Design review of the part built by this model. Coordinates are the model's own, in mm. A direction names the side the tool comes from. Round coordinates to 2 decimals unless told otherwise and drop trailing zeros. Loops run counter-clockwise (first coordinate to the right, second up) from the corner with the lowest first, then second, coordinate; pieces in that order, holes last. Notation, with made-up numbers: (-39.5, -7) - (4.5, -7) arc R26 cw to (4.5, 29) - close; hole circle Ø2 at (-14, 64). An arc over 180 degrees is marked (long way). Answer as CSV lines item,"result". Start each with the question number.
(1) Consider section C-C (x = 9.75). Give the boundary of the cut face in (y, z).
(2) For P1, Ø2, axis at y = -31, z = -8.5, coming from the +X side; P2, Ø6.5, axis at x = 11, z = -7.5, coming from the +Y side; P3, Ø10, axis at x = 15, y = -48.5, coming from the -Z side, all flat-tipped, find the tip position at first contact; note any pin that passes through.
(3) Consider section A-A (x = 15.4). Give the boundary of the cut face in (y, z).
(4) Mouldability with a two-part tool opening along X and no side actions: class faces 1 (the flat face through (14, -52.511, -3)), 2 (the cylindrical face through (3.417, -42.54, -3.588)), 3 (the flat face through (0, -20, -10)) as released by +X, released by -X, zero draft, split by the parting line, or undercut.
(5) Consider section B-B (y = -42.8). Give the boundary of the cut face in (x, z) (3 decimals), and give its area (3 significant figures).
(6) Wall thickness on L1, parallel to X at y = -42.8, z = -3.25 (3 decimals); L2, parallel to Y at x = 15.4, z = -2.75; L3, parallel to Y at x = 10.75, z = -5: over which ranges is each line inside the solid? List them lowest first.
(7) For faces 4 (the flat face through (-2, -20, 0)), 5 (the flat face through (13, 6, -6.35)), 6 (the flat face through (14, 12.7, -3)), 7 (the flat face through (-2, -21, -19.05)), 8 (the flat face through (10, 0, -3)), list the 3-axis set-ups (+Z, -Z, +X, -X, +Y, -Y) from which the entire face can be reached by the end or side of a thin tool; tool diameter is ignored.
(8) Consider section D-D (z = -3.5). Give the boundary of the cut face in (x, y) (3 decimals).
Autodesk Inventor part; units mm, degrees
ref_plane "YZ Plane" through (0, 0, 0) normal (1, 0, 0) x (0, 1, 0)
ref_plane "XZ Plane" through (0, 0, 0) normal (0, 1, 0) x (-1, 0, 0)
ref_plane "XY Plane" through (0, 0, 0) normal (0, 0, 1) x (1, 0, 0)
sketch "Sketch1" plane through (0, 0, 0) normal (0, 0, 1) x (1, 0, 0)
  line L0 (0, 0) -> (20.8, 0)
  line L1 (20.8, 0) -> (20.8, 12.7)
  line L2 (20.8, 12.7) -> (0, 12.7)
  line L3 (0, 12.7) -> (0, 0)
  line L4 (0, -39.8112) -> (20.8, -39.8112)
  line L5 (20.8, -39.8112) -> (20.8, -52.5112)
  line L6 (20.8, -52.5112) -> (0, -52.5112)
  line L7 (0, -52.5112) -> (0, -39.8112)
  line L8 (10.4, 12.7) -> (10.4, 0)
  point P0 (5.4, 3)
  dimension "d0" = 20.8
  dimension "d1" = 12.7
  dimension "d2" = 39.8112
  dimension "d33" = 3
  dimension "d34" = 5
  dimension "d41" = 10.4
extrude "Extrusion1" add sketch "Sketch1" against normal blind 6.35
hole "Hole3" at (5.4, 3, 0) direction (0, 0, -1) diameter 4 depth 25.4
pattern_linear "Rectangular Pattern1" count 2 spacing 10 along (1, 0, 0) count 2 spacing 45.8 along (0, -1, 0) of "Hole3"
sketch "Sketch3" plane through (0, 0, 0) normal (-1, 0, 0) x (0, 0, 1)
  line L0 (0, 12.7) -> (0, 0)
  line L1 (-19.05, 24.4) -> (0, 24.4)
  line L2 (0, 24.4) -> (0, -65.2112)
  line L3 (0, -65.2112) -> (-19.05, -65.2112)
  line L4 (-19.05, -65.2112) -> (-19.05, 24.4)
  line L5 (0, -39.8112) -> (-6.35, -39.8112)
  dimension "d42" = 19.05
  dimension "ServoMountLength" = 89.6112
  dimension "d45" = 25.4
extrude "Extrusion2" add sketch "Sketch3" along normal blind 3.175
fillet "Fillet1" radius 6.35 4 edges at (0, 6.35, -6.35) (0, 12.7, -3.175) (0, -46.1612, -6.35) (0, -52.5112, -3.175)
equation "\"d0\" = ServoWidth + ServoTolerance"
equation "\"d2\" = ServoLength + ServoTolerance"
equation "\"d41\" = 0.5 * ServoTolerance + 0.5 * ServoWidth"
equation "\"d37\" = ServoScrewSpacing"
equation "\"d40\" = ServoScrewSpacingLength"
equation "\"ServoTolerance\" = 1"
properties part number "ServoMount" material "ABS Plastic"
Determined:
1,outline,"(-52.51, -6.35) - (-39.81, -6.35) - (-39.81, 0) - (-52.51, 0) - close; (0, -6.35) - (12.7, -6.35) - (12.7, 0) - (0, 0) - close"
2,P1,"stops at x = 0"
2,P2,"stops at y = 12.7"
2,P3,"stops at z = -6.35"
3,outline,"(-52.51, -6.35) - (-44.8, -6.35) - (-44.8, 0) - (-52.51, 0) - close; (-40.8, -6.35) - (-39.81, -6.35) - (-39.81, 0) - (-40.8, 0) - close; (0, -6.35) - (1, -6.35) - (1, 0) - (0, 0) - close; (5, -6.35) - (12.7, -6.35) - (12.7, 0) - (5, 0) - close"
4,face 1,"zero draft"
4,face 2,"undercut"
4,face 3,"released by +X"
5,outline,"(-3.175, -19.05) - (0, -19.05) - (0, -12.7) arc R6.35 cw to (3.4, -7.077) - (3.4, 0) - (-3.175, 0) - close; (7.4, -6.35) - (13.4, -6.35) - (13.4, 0) - (7.4, 0) - close; (17.4, -6.35) - (20.8, -6.35) - (20.8, 0) - (17.4, 0) - close"
5,area,"150 mm^2"
6,L1,"x = -3.175 to 3.4, 7.4 to 13.4, 17.4 to 20.8"
6,L2,"y = -52.51 to -44.8, -40.8 to -39.81, 0 to 1, 5 to 12.7"
6,L3,"y = -52.51 to -39.81, 0 to 12.7"
7,face 4,"+Z, +X, -X, +Y, -Y"
7,face 5,"-Z, +X, +Y, -Y"
7,face 6,"+Z, -Z, +X, +Y"
7,face 7,"-Z, +X, -X, +Y, -Y"
7,face 8,"+Z, -Z, +X"
8,outline,"(-3.175, -65.211) - (0, -65.211) - (0, -58.861) arc R6.35 cw to (6.35, -52.511) - (20.8, -52.511) - (20.8, -39.811) - (0, -39.811) - (0, 0) - (20.8, 0) - (20.8, 12.7) - (6.35, 12.7) arc R6.35 cw to (0, 19.05) - (0, 24.4) - (-3.175, 24.4) - close; hole circle Ø4 at (5.4, -42.8); hole circle Ø4 at (5.4, 3); hole circle Ø4 at (15.4, -42.8); hole circle Ø4 at (15.4, 3)"
